Here's how the part is built. I have some questions about the finished solid (model axes, mm). A direction names the side the tool comes from. Coordinates: 2 decimals unless noted, no trailing zeros. Write each loop counter-clockwise with the first axis right and the second up, starting at its lowest first coordinate (ties: lowest second). Pieces come first, ordered by that corner, then holes.
from build123d import *

# Parameters (mm, degrees)
SKETCH1_W           = 40
SKETCH1_H           = 21
BOSS_EXTRUDE1_DEPTH = 3
SKETCH2_W           = 40
SKETCH2_H           = 3
BOSS_EXTRUDE2_DEPTH = 3
SKETCH3_W           = 22.2
SKETCH3_H           = 11.8
CUT_EXTRUDE1_DEPTH  = 10
SKETCH4_R           = 1.5
CUT_EXTRUDE2_DEPTH  = 10


with BuildPart() as part:
    # Sketch1 → Boss-Extrude1 (new body)
    with BuildSketch(Plane(origin=(0, 0, 0), x_dir=(1, 0, 0), z_dir=(0, 1, 0))):
        with Locations((20, 10.5)):
            Rectangle(SKETCH1_W, SKETCH1_H)
    extrude(amount=BOSS_EXTRUDE1_DEPTH)

    # Sketch2 → Boss-Extrude2 (add)
    with BuildSketch(Plane(origin=(0, 0, -21), x_dir=(-1, 0, 0), z_dir=(0, 0, -1))):
        with Locations((-20, 1.5)):
            Rectangle(SKETCH2_W, SKETCH2_H)
    extrude(amount=BOSS_EXTRUDE2_DEPTH)

    # Sketch3 → Cut-Extrude1 (cut)
    with BuildSketch(Plane(origin=(0, 3, 0), x_dir=(1, 0, 0), z_dir=(0, 1, 0))):
        with Locations((23.9, 15.1)):
            Rectangle(SKETCH3_W, SKETCH3_H)
    extrude(amount=-CUT_EXTRUDE1_DEPTH, mode=Mode.SUBTRACT)

    # Sketch4 → Cut-Extrude2 (cut)
    with BuildSketch(Plane(origin=(0, 3, 0), x_dir=(1, 0, 0), z_dir=(0, 1, 0))):
        with Locations(Location((10.3, 15.1, 0), (0, 0, 270))):
            Circle(SKETCH4_R)
        with Locations(Location((37.5, 15.1, 0), (0, 0, 270))):
            Circle(SKETCH4_R)
    extrude(amount=-CUT_EXTRUDE2_DEPTH, mode=Mode.SUBTRACT)


solid = part.part
1. I want a section at B-B (x = 15). List the corners of the cut face in (y, z) for me, then the cut area to 3 significant figures.
2. If I drill on line 1 (X direction, y = 1.85, z = -15.1); line 2 (X direction, y = 1, z = -13); line 3 (Z direction, x = 25.5, y = 2.45), over which ranges is the centre line in solid material (lowest first)?
3. For pin 1 Ø3 at (x, z) = (5.5, -4.5) entering from -Y, with a flat end and sliding along its axis, tell me the tip position at first contact or that it passes through.
4. I want a section at C-C (z = -15.1). List the corners of the cut face in (x, y) for me, then the cut area to 3 significant figures.
5. I want a section at D-D (y = 2.2). List the corners of the cut face in (x, z) for me.
6. I want a section at A-A (z = -10.5). List the corners of the cut face in (x, y) for me.
7. On a 3-axis mill with a long thin cutter (end or side, diameter ignored), from which of +Z, -Z, +X, -X, +Y, -Y can I reach the whole of each face in a straight line? I mean faces 1 (the face through (20, 1, 0)), 2 (the face through (24, 2, -9.2)). Say none if no direction works.
Response values:
1. outline: (0, -24) - (3, -24) - (3, -21) - (0, -21) - close; (0, -9.2) - (3, -9.2) - (3, 0) - (0, 0) - close
1. area: 36.6 mm2
2. line 1: x = 0 to 8.8, 11.8 to 12.8, 35 to 36, 39 to 40
2. line 2: x = 0 to 12.8, 35 to 40
2. line 3: z = -24 to -21, -9.2 to 0
3. pin 1: stops at y = 0
4. outline: (0, 0) - (8.8, 0) - (8.8, 3) - (0, 3) - close; (11.8, 0) - (12.8, 0) - (12.8, 3) - (11.8, 3) - close; (35, 0) - (36, 0) - (36, 3) - (35, 3) - close; (39, 0) - (40, 0) - (40, 3) - (39, 3) - close
4. area: 35.4 mm2
5. outline: (0, -24) - (40, -24) - (40, 0) - (0, 0) - close; hole circle Ø3 at (10.3, -15.1); hole (12.8, -21) - (35, -21) - (35, -9.2) - (12.8, -9.2) - close; hole circle Ø3 at (37.5, -15.1)
6. outline: (0, 0) - (12.8, 0) - (12.8, 3) - (0, 3) - close; (35, 0) - (40, 0) - (40, 3) - (35, 3) - close
7. face 1: +Z, +X, -X, +Y, -Y
7. face 2: +Y, -Y
